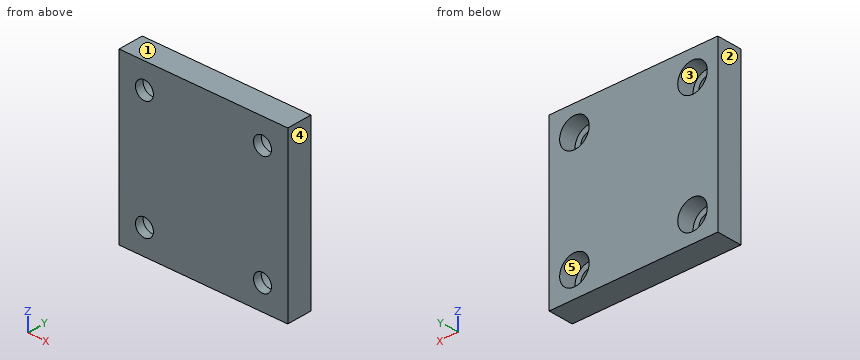
Autodesk Inventor part; units mm, degrees
ref_plane "YZ Plane" through (0, 0, 0) normal (1, 0, 0) x (0, 1, 0)
ref_plane "XZ Plane" through (0, 0, 0) normal (0, 1, 0) x (-1, 0, 0)
ref_plane "XY Plane" through (0, 0, 0) normal (0, 0, 1) x (1, 0, 0)
sketch "Sketch1" plane through (0, 0, 0) normal (0, 1, 0) x (-1, 0, 0)
  line L0 (0, 0) -> (-63.5, 0)
  line L1 (-63.5, 0) -> (-63.5, -63.5)
  line L2 (-63.5, -63.5) -> (0, -63.5)
  line L3 (0, -63.5) -> (0, 0)
  dimension "d0" = 63.5
  dimension "d1" = 63.5
extrude "Extrusion1" add sketch "Sketch1" along normal blind 9.525
sketch "Sketch2" plane through (0, 9.525, 0) normal (0, 1, 0) x (1, 0, 0)
  line L0 (0, 0) -> (63.5, 0)
  line L1 (63.5, 0) -> (63.5, 63.5)
  line L2 (63.5, 63.5) -> (0, 63.5)
  line L3 (0, 63.5) -> (0, 0)
  line L4 (9.525, 53.975) -> (53.975, 53.975)
  line L5 (53.975, 53.975) -> (53.975, 9.525)
  line L6 (53.975, 9.525) -> (9.525, 9.525)
  line L7 (9.525, 9.525) -> (9.525, 53.975)
  dimension "d4" = 9.525
hole "Hole1" at (53.975, 9.525, -9.525) at (53.975, 9.525, -53.975) at (9.525, 9.525, -53.975) at (9.525, 9.525, -9.525) direction (0, -1, 0) diameter 6.7564 end through all counterbore diameter 11.1252 counterbore depth 6.35
equation "\"d0\" = d1"
properties part number "Block"
CAD build for the part. Positions are in the model's coordinates, mm. Face numbers are marked on the shaded views. A direction names the side the tool comes from. Give positions to 0.01 mm unless a question says otherwise; leave off trailing zeros. Write each loop counter-clockwise with the first axis right and the second up, starting at its lowest first coordinate (ties: lowest second). Pieces come first, ordered by that corner, then holes. Notation, with made-up numbers: M -17.5,77.5 L 19.5,77.5 A9 ccw 19.5,84.5 Z; hole C 35.25,69.25 d1. An arc over 180 degrees is marked long. Return JSON: item names as keys, results as strings. Group by question number.
(1) Mould opens along X. For the marked faces 1, 2 and 3 say: pulls with the +X half, pulls with the -X half, needs draft (parallel to the pull), parting line crosses it, or undercut.
(2) 3-axis set-ups, long thin cutter, end or side, ignore diameter. For the marked faces 4 and 5: which of +Z, -Z, +X, -X, +Y, -Y reach the whole face in a straight line?
(3) Band-saw the part on A-A (y = 8.25). Give the cut face in (x, z) (3 decimals).
(4) Flat gauge pins, fed straight in: pin 1 Ø6.5 at (x, z) = (9.525, -53.975) entering from +Y; pin 2 Ø9 at (x, z) = (53.5, -53.5) entering from +Y (3 decimals). Where does each tip first touch, or does it go through?
(5) Band-saw the part on C-C (x = 52). Give the cut face in (y, z) (3 decimals), and give its area (3 significant figures).
(6) Band-saw the part on B-B (x = 14). Give the cut face in (y, z) (3 decimals), and give its area (3 significant figures).
(7) Drill centre lines: L1, parallel to X at y = 5, z = -55; L2, parallel to X at y = 7, z = -13; L3, parallel to Z at x = 52.5, y = 5.5. Where is each one in solid material? Low to high. Write a range as [from, to].
(8) Band-saw the part on D-D (y = 1.75). Give the cut face in (x, z) (3 decimals).
Entries:
{
 "1": {"face 1": "needs draft", "face 2": "pulls with the -X half", "face 3": "undercut"},
 "2": {"face 4": "+Z, -Z, +X, +Y, -Y", "face 5": "+Y"},
 "3": {"outline": "M 0,-63.5 L 63.5,-63.5 L 63.5,0 L 0,0 Z; hole C 9.525,-53.975 d11.125; hole C 9.525,-9.525 d11.125; hole C 53.975,-53.975 d11.125; hole C 53.975,-9.525 d11.125"},
 "4": {"pin 1": "passes through", "pin 2": "stops at y = 3.175"},
 "5": {"outline": "M 0,-63.5 L 9.525,-63.5 L 9.525,-59.175 L 3.175,-59.175 L 3.175,-56.716 L 0,-56.716 Z; M 0,-51.234 L 3.175,-51.234 L 3.175,-48.775 L 9.525,-48.775 L 9.525,-14.725 L 3.175,-14.725 L 3.175,-12.266 L 0,-12.266 Z; M 0,-6.784 L 3.175,-6.784 L 3.175,-4.325 L 9.525,-4.325 L 9.525,0 L 0,0 Z", "area": "438 mm^2"},
 "6": {"outline": "M 0,-63.5 L 9.525,-63.5 L 9.525,-57.279 L 3.175,-57.279 L 3.175,-50.671 L 9.525,-50.671 L 9.525,-12.829 L 3.175,-12.829 L 3.175,-6.221 L 9.525,-6.221 L 9.525,0 L 0,0 Z", "area": "521 mm^2"},
 "7": {"L1": "x = [0, 4.06], [14.99, 48.51], [59.44, 63.5]", "L2": "x = [0, 5.18], [13.87, 49.63], [58.32, 63.5]", "L3": "z = [-63.5, -59.34], [-48.61, -14.89], [-4.16, 0]"},
 "8": {"outline": "M 0,-63.5 L 63.5,-63.5 L 63.5,0 L 0,0 Z; hole C 9.525,-53.975 d6.756; hole C 9.525,-9.525 d6.756; hole C 53.975,-53.975 d6.756; hole C 53.975,-9.525 d6.756"}
}
